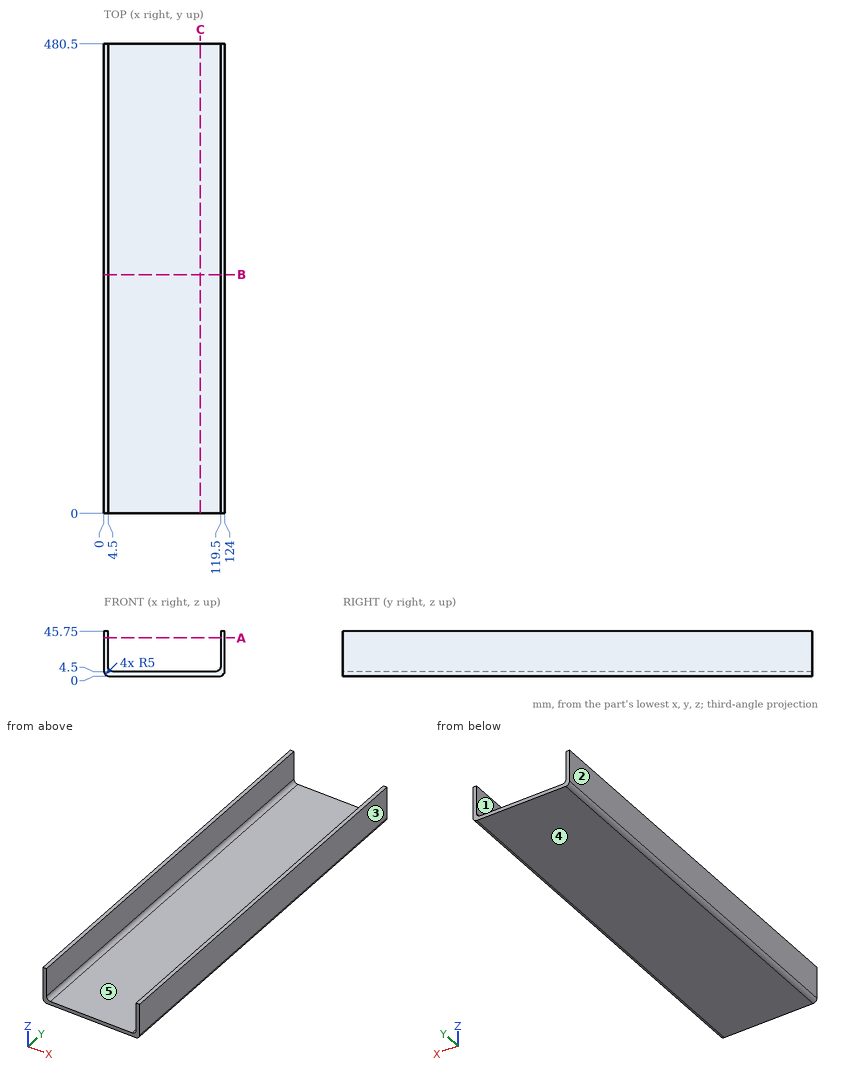
Source: three-view drawing plus pictorial views. Frame: mm from the lowest corner of the part. A direction names the side the tool comes from. Round coordinates to 2 decimals unless told otherwise and drop trailing zeros. Loops run counter-clockwise (first coordinate to the right, second up) from the corner with the lowest first, then second, coordinate; pieces in that order, holes last. Notation, with made-up numbers: (70.25, 68.5) - (104.25, 68.5) arc R27 cw to (104.25, 92.5) - close; hole circle Ø6 at (63.5, 65). An arc over 180 degrees is marked (long way). Write item = value, one per line. Start each with the question number.
Item 1: Section query B-B on y = 244.5. Output: boundary loops of the cut face in (x, z).
Item 2: First-contact query: pin 1 Ø3 at (x, y) = (33, 318) entering from +Z. Flat tip, straight axial feed; report the tip coordinate or a pass-through.
Item 3: Section query A-A on z = 39. Output: boundary loops of the cut face in (x, y).
Item 4: Material intervals for line 1 (X direction, y = 281, z = 21); line 2 (Z direction, x = 62, y = 110.5); line 3 (X direction, y = 273, z = 3.5), sorted ascending.
Item 5: Section query C-C on x = 99. Output: boundary loops of the cut face in (y, z).
Item 6: Mould query, pull axis X, two halves, no side actions, for the marked faces 1, 2 and 3. Classes: released by +X, released by -X, zero draft, split by the parting line, or undercut.
Item 7: Reachability of the marked faces 4 and 5 from +Z, -Z, +X, -X, +Y, -Y: full face, straight path, thin tool, end or side. Return the list, or none.
Results list:
q1.outline = (0, 5) arc R5 ccw to (5, 0) - (119, 0) arc R5 ccw to (124, 5) - (124, 45.75) - (119.5, 45.75) - (119.5, 9.5) arc R5 cw to (114.5, 4.5) - (9.5, 4.5) arc R5 cw to (4.5, 9.5) - (4.5, 45.75) - (0, 45.75) - close
q2.pin_1 = 4.5
q3.outline = (0, 0) - (4.5, 0) - (4.5, 480.5) - (0, 480.5) - close; (119.5, 0) - (124, 0) - (124, 480.5) - (119.5, 480.5) - close
q4.line_1 = 0 to 4.5, 119.5 to 124
q4.line_2 = 0 to 4.5
q4.line_3 = 0.23 to 123.77
q5.outline = (0, 0) - (480.5, 0) - (480.5, 4.5) - (0, 4.5) - close
q6.face_1 = undercut
q6.face_2 = released by -X
q6.face_3 = released by +X
q7.face_4 = -Z, +X, -X, +Y, -Y
q7.face_5 = +Z, +Y, -Y
